Autodesk Inventor part; units mm, degrees
ref_plane "Płaszczyzna konstrukcyjna1" through (0, -12, 0) normal (0, 0, -1) x (-1, 0, 0)
ref_plane "Płaszczyzna konstrukcyjna2" through (0, -10, -2.2657) normal (1, 0, 0) x (0, 0, -1)
ref_plane "YZ Plane" through (0, 0, 0) normal (1, 0, 0) x (0, 1, 0)
sketch "Szkic1" plane through (0, 0, 0) normal (0, 1, 0) x (-1, 0, 0)
  circle A0 centre (0, 0) radius 12.5
  circle A1 centre (0, 0) radius 10
  dimension "d0" = 20
  dimension "d2" = 25
extrude "Wyciągnięcie proste1" add sketch "Szkic1" along normal blind 5
ref_plane "Płaszczyzna konstrukcyjna1" through (0, -12, 0) normal (0, 0, -1) x (-1, 0, 0)
sketch "Szkic5" plane through (0, -12, 0) normal (0, 0, -1) x (-1, 0, 0)
  line L0 (12.5, 17) -> (-12.5, 17)
  line L1 (0, 17) -> (-12.5, 17)
  line L2 (-12.5, 17) -> (-12.5, 18.75)
  line L3 (-12.5, 18.75) -> (0, 18.75)
  line L4 (0, 18.75) -> (0, 17)
  line L5 (0, 18.75) -> (-9.5, 18.75)
  line L6 (-9.5, 18.75) -> (-9.5, 21.25)
  line L7 (-9.5, 21.25) -> (0, 21.25)
  line L8 (0, 21.25) -> (0, 18.75)
  line L9 (0, 21.25) -> (-12.5, 21.25)
  line L10 (-12.5, 21.25) -> (-12.5, 23)
  line L11 (-12.5, 23) -> (0, 23)
  line L12 (0, 23) -> (0, 21.25)
  line L13 (0, 23) -> (-9.5, 23)
  line L14 (-9.5, 23) -> (-9.5, 25.5)
  line L15 (-9.5, 25.5) -> (0, 25.5)
  line L16 (0, 25.5) -> (0, 23)
  line L17 (0, 25.5) -> (-12.5, 25.5)
  line L18 (-12.5, 25.5) -> (-12.5, 27.25)
  line L19 (-12.5, 27.25) -> (0, 27.25)
  line L20 (0, 27.25) -> (0, 25.5)
  line L21 (0, 27.25) -> (-9.5, 27.25)
  line L22 (-9.5, 27.25) -> (-9.5, 29.75)
  line L23 (-9.5, 29.75) -> (0, 29.75)
  line L24 (0, 29.75) -> (0, 27.25)
  line L25 (0, 29.75) -> (-12.5, 29.75)
  line L26 (-12.5, 29.75) -> (-12.5, 31.5)
  line L27 (-12.5, 31.5) -> (0, 31.5)
  line L28 (0, 31.5) -> (0, 29.75)
  line L29 (-12.5, 12) -> (-12.5, 17) construction
  line L30 (-12.5, 12) -> (-12.5, 17) construction
  line L31 (-12.5, 12) -> (12.5, 12) construction
  point P0 (0, 12)
  dimension "d13" = 2.5
  dimension "d17" = 19.5
  dimension "d18" = 3
revolve "Obrót1" add sketch "Szkic5" angle 360 about axis through (0, 11, 0) along (0, -1, 0)
sketch "Szkic7" plane through (0, 17.75, 0) normal (0, -1, 0) x (1, 0, 0)
  circle A0 centre (0, 0) radius 9.5
  circle A1 centre (0, 9.5) radius 1.65
  circle A2 centre (0, 0) radius 10
  circle A3 centre (0, 0) radius 9.5
  circle A4 centre (-9.5, 0) radius 1.65
  circle A5 centre (0, -9.5) radius 1.65
  circle A6 centre (9.5, 0) radius 1.65
  circle A7 centre (6.7175, -6.7175) radius 0.9
  circle A8 centre (6.7175, 6.7175) radius 0.9
  circle A9 centre (-6.7175, 6.7175) radius 0.9
  circle A10 centre (-6.7175, -6.7175) radius 0.9
  line L0 (6.7175, 6.7175) -> (0, 0) construction
  line L1 (0, 0) -> (-6.7175, 6.7175) construction
  circle A11 centre (0, 0) radius 12.5 construction
  line L2 (0, 0) -> (-6.7175, -6.7175) construction
  line L3 (0, 0) -> (6.7175, -6.7175) construction
  line L4 (17.5, 0) -> (-17.5, 0) construction
  dimension "d23" = 45
  dimension "d24" = 45
  dimension "d25" = 3.3
  dimension "d47" = 1.8
extrude "Wyciągnięcie proste6" cut sketch "Szkic7" along normal up to surface (11 mm away) contours A0 A6 | A0 A6 A2 | A8 A0 | A0 A8 A2 | A6 A2 | A7 A2 A0 | A0 A7 | A2 A8 | A7 A2 | A1 A0 | A0 A1 A2 | A5 A2 A0 | A0 A5 | A2 A1 | A5 A2 | A9 A0 | A0 A9 A2 | A10 A2 A0 | A0 A10 | A2 A9 | A10 A2 | A4 A0 | A0 A4 A2 | A2 A4
sketch "Szkic8" plane through (0, -12, 0) normal (0, 0, -1) x (-1, 0, 0)
  line L0 (6.0517, 25.5) -> (1.6438, 25.5)
  line L1 (-1.6438, 25.5) -> (-1.6438, 23)
  line L2 (1.6438, 25.5) -> (-1.6438, 25.5)
  line L3 (-1.6438, 25.5) -> (-1.6438, 23)
  line L4 (-1.6438, 23) -> (1.6438, 23)
  line L5 (1.6438, 23) -> (1.6438, 25.5)
  point P0 (0, 12)
  point P1 (1.65, 22.75)
extrude "Wyciągnięcie proste7" cut sketch "Szkic8" along normal through all both and the other way through all
sketch "Szkic9" plane through (0, 5, 0) normal (0, -1, 0) x (1, 0, 0)
  line L0 (0, 0) -> (-3.4352, 0)
  line L1 (-3.4352, 0) -> (-3.4352, -2.2657)
  line L2 (-3.4352, -2.2657) -> (0, -2.2657)
  line L3 (0, -2.2657) -> (0, 0)
  dimension "d30" = 3.4352
  dimension "d31" = 2.2658
extrude "Wyciągnięcie proste8" add sketch "Szkic9" along normal blind 15
ref_plane "Płaszczyzna konstrukcyjna2" through (0, -10, -2.2657) normal (1, 0, 0) x (0, 0, -1)
sketch "Szkic10" plane through (0, -10, 0) normal (0, -1, 0) x (1, 0, 0)
  line L0 (0, 0) -> (-3.4352, 0)
  line L1 (-3.4352, -2.2657) -> (0, -2.2657)
  line L2 (0, 0) -> (-3.4352, 0)
  line L3 (-3.4352, 0) -> (-3.4352, -2.2657)
  line L4 (-3.4352, -2.2657) -> (0, -2.2657)
  line L5 (0, -2.2657) -> (0, 0)
extrude "Wyciągnięcie proste9" cut sketch "Szkic10" against normal up to surface (15 mm away)
sketch "Szkic11" plane through (0, -10, -2.2657) normal (1, 0, 0) x (0, 0, -1)
  line L0 (-3.9095, 21) -> (-3.9095, 23.5)
  line L1 (-0.622, 21) -> (-0.622, 23.5)
  line L2 (-3.9095, 21) -> (-0.622, 21)
  line L3 (-0.622, 21) -> (-0.622, 23.5)
  line L4 (-0.622, 23.5) -> (-3.9095, 23.5)
  line L5 (-3.9095, 23.5) -> (-3.9095, 21)
  point P0 (-2.2657, 10)
extrude "Wyciągnięcie proste10" cut sketch "Szkic11" along normal through all both and the other way through all
sketch "Szkic12" plane through (0, 19.5, 0) normal (0, 1, 0) x (1, 0, 0)
  line L0 (0, 0) -> (4.6374, 4.6374) construction
  line L1 (0, 0) -> (6.5583, 0) construction
  line L2 (0, 0) -> (-4.6374, 4.6374) construction
  line L3 (0, 0) -> (-4.8503, -4.8503) construction
  line L4 (0, 0) -> (4.8503, -4.8503) construction
  point P0 (-4.6374, 4.6374)
  point P1 (4.6328, -4.7775)
  dimension "d39" = 6.5583
hole "Otwór1" at (4.6374, 19.5, -4.6374) at (-4.6374, 19.5, -4.6374) at (-4.8503, 19.5, 4.8503) at (4.6328, 19.5, 4.7775) direction (0, -1, 0) diameter 3.4 end through all countersink diameter 6.9 countersink angle 89.954
properties part number "Koło2"
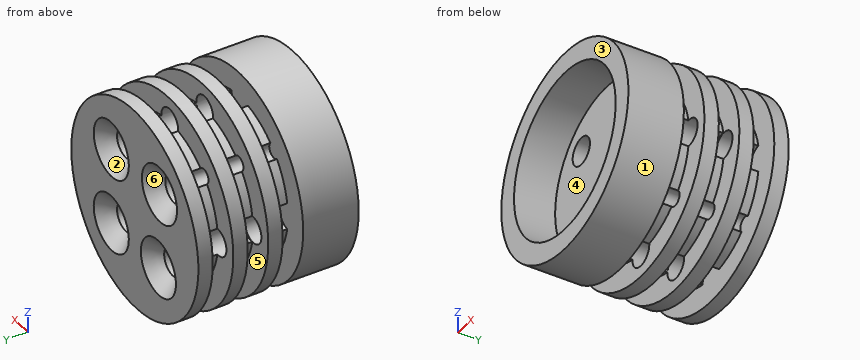
Could you check a few things on this model? Use its own coordinates, in mm. Face numbers are marked on the shaded views. A direction names the side the tool comes from. Round coordinates to 2 decimals unless told otherwise and drop trailing zeros. Order: outer loops, then holes, each group sorted by start corner. A loop starts at its lowest first (then second) coordinate and runs counter-clockwise, first axis right, second up.
(1) Please list where these lines run through material, in increasing order: line 1 along Z through (x, y) = (0, 15.15); line 2 along X through (y, z) = (14.25, -5.25); line 3 along Z through (x, y) = (0, 3.3).
Response values:
line 1: z = -12.5 to -11.15, -7.85 to 7.85, 11.15 to 12.5
line 2: x = -11.34 to -6.22, -3.05 to 3.05, 6.22 to 11.34
line 3: z = -12.5 to -10, 10 to 12.5
(2) I'm going to push flat-ended pins straight in: pin 1 (6 mm diameter, centred on y = 10, z = -5.5, fed in from -X); pin 2 (3 mm diameter, centred on x = 5, y = 12, fed in from +Z); pin 3 (12.5 mm diameter, centred on x = -2, z = 1, fed in from -Y). Where does each tip first touch, or does it pass through?
Response values:
pin 1: stops at x = -12.25
pin 2: stops at z = 11.88
pin 3: stops at y = 5
(3) Which directions (+Z, -Z, +X, -X, +Y, -Y) give clear straight access to the entire face, cutting with the end or side of a thin tool? Please do the marked faces 4, 5 and 6.
Response values:
face 4: -Y
face 5: none
face 6: +Y
(4) Imagine slicing it at D-D (y = 3.75). Write out the boundary of the cut face in (x, z), plus the area to 3 significant figures.
Response values:
outline: circle Ø25 at (0, 0); hole circle Ø20 at (0, 0)
area: 177 mm2
(5) Imagine slicing it at A-A (y = 11.5). Count the separate pieces of the cut face and the enclosed holes in it, plus the area to 3 significant figures.
Response values:
separate pieces: 4
enclosed holes: 4
area: 129 mm2
(6) If we mould it in two halves opening along X, with no side actions, what happens to the marked faces 1, 2 and 3? For each: released by +X, released by -X, zero draft, split by the parting line, or undercut.
Response values:
face 1: split by the parting line
face 2: undercut
face 3: zero draft
